For this review, take the finished solid that the model builds, in its own axes (mm). Face numbers are marked on the shaded views. Round coordinates to 2 decimals unless told otherwise and drop trailing zeros. Order: outer loops, then holes, each group sorted by start corner. A loop starts at its lowest first (then second) coordinate and runs counter-clockwise, first axis right, second up. Notation, with made-up numbers: (-36.5, 52) -> (-13.5, 52) arc R15 ccw to (-13.5, 71) -> close; hole circle Ø8 at (-5, -26). An arc over 180 degrees is marked (long way). Put each result on its own line as item: value. Start each with the question number.
```python
from build123d import *

# Parameters (mm, degrees)
BOSS_EXTRUDE1_DEPTH = 50
SKETCH2_R           = 2.5
CUT_EXTRUDE1_DEPTH  = 5


with BuildPart() as part:
    # Sketch1 → Boss-Extrude1 (new body)
    with BuildSketch(Plane(origin=(0, 0, 0), x_dir=(0, 0, -1), z_dir=(1, 0, 0))):
        with BuildLine():
            Line((24, -16.5), (9.19407636, -16.5))
            Line((9.19407636, -16.5), (7.575142847, -13.028185878))
            ThreePointArc((7.575142847, -13.028185878), (0, 3.5), (-7.575142847, -13.028185878))
            Line((-7.575142847, -13.028185878), (-9.19407636, -16.5))
            Line((-9.19407636, -16.5), (-24, -16.5))
            Line((-24, -16.5), (-24, 16.5))
            Line((-24, 16.5), (24, 16.5))
            Line((24, 16.5), (24, -16.5))
        make_face()
    extrude(amount=BOSS_EXTRUDE1_DEPTH)

    # Sketch2 → Cut-Extrude1 (cut)
    with BuildSketch(Plane(origin=(0, 16.5, 0), x_dir=(1, 0, 0), z_dir=(0, 1, 0))):
        with Locations((7.5, 17.5)):
            Circle(SKETCH2_R)
        with Locations((42.5, 17.5)):
            Circle(SKETCH2_R)
        with Locations((42.5, -17.5)):
            Circle(SKETCH2_R)
        with Locations((7.5, -17.5)):
            Circle(SKETCH2_R)
    extrude(amount=-CUT_EXTRUDE1_DEPTH, mode=Mode.SUBTRACT)


solid = part.part
```
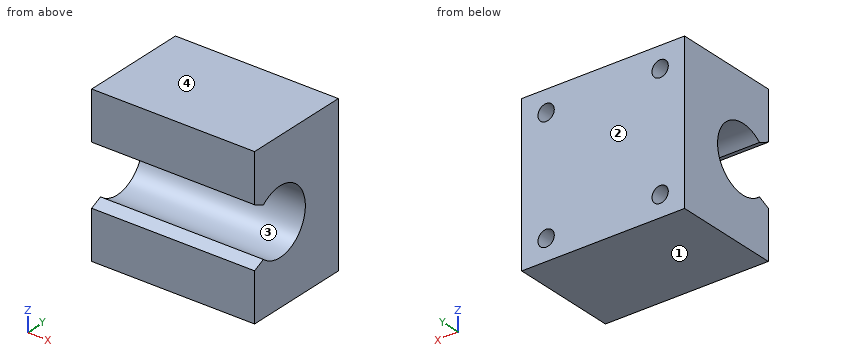
Item 1: Consider section B-B, the plane z = -17.5. Write out the cut boundary in (x, y), plus the area to 3 significant figures.
Item 2: For L1, parallel to Z at x = 42.5, y = 12.7; L2, parallel to X at y = 15.3, z = 17.5; L3, parallel to X at y = 12, z = 17, list the stretches that pass through material, from the lowest coordinate up.
Item 3: Consider section D-D, the plane y = 13.5. Write out the cut boundary in (x, z), plus the area to 3 significant figures.
Item 4: Consider section C-C, the plane x = 42.5. Write out the cut boundary in (y, z).
Item 5: Consider section A-A, the plane y = -6.5. Write out the cut boundary in (x, z).
Item 6: Insertion check: pin 1 Ø16 at (y, z) = (-6.5, 0) entering from +X; pin 2 Ø6 at (x, z) = (16, -1) entering from -Y; pin 3 Ø1.5 at (x, z) = (41.5, 17) entering from +Y. Each pin has a flat end and moves straight along its axis. Give the tip position at first contact, or say it passes through.
Item 7: Mouldability with a two-part tool opening along Z and no side actions: class the marked faces 1, 2, 3 and 4 as +Z half, -Z half, draft (parallel to the pull), parting line (faces both ways), or undercut.
Evaluation:
1. outline: (0, -16.5) -> (50, -16.5) -> (50, 16.5) -> (45, 16.5) -> (45, 11.5) -> (40, 11.5) -> (40, 16.5) -> (10, 16.5) -> (10, 11.5) -> (5, 11.5) -> (5, 16.5) -> (0, 16.5) -> close
1. area: 1,600 mm^2
2. L1: z = -24 to -20, -15 to 15, 20 to 24
2. L2: x = 0 to 5, 10 to 40, 45 to 50
2. L3: x = 0 to 5.05, 9.95 to 40.05, 44.95 to 50
3. outline: (0, -24) -> (50, -24) -> (50, 24) -> (0, 24) -> close; hole circle Ø5 at (7.5, -17.5); hole circle Ø5 at (7.5, 17.5); hole circle Ø5 at (42.5, -17.5); hole circle Ø5 at (42.5, 17.5)
3. area: 2,320 mm^2
4. outline: (-16.5, -24) -> (16.5, -24) -> (16.5, -20) -> (11.5, -20) -> (11.5, -15) -> (16.5, -15) -> (16.5, 15) -> (11.5, 15) -> (11.5, 20) -> (16.5, 20) -> (16.5, 24) -> (-16.5, 24) -> (-16.5, 9.19) -> (-13.03, 7.58) arc R10 cw (long way) to (-13.03, -7.58) -> (-16.5, -9.19) -> close
5. outline: (0, -24) -> (50, -24) -> (50, -10) -> (0, -10) -> close; (0, 10) -> (50, 10) -> (50, 24) -> (0, 24) -> close
6. pin 1: passes through
6. pin 2: stops at y = 2.67
6. pin 3: stops at y = 11.5
7. face 1: -Z half
7. face 2: draft
7. face 3: undercut
7. face 4: +Z half
